from build123d import *

# Parameters (mm, degrees)
SKETCH1_R           = 10
BOSS_EXTRUDE1_DEPTH = 5
BOSS_EXTRUDE2_DEPTH = 125
SKETCH3_W           = 50
SKETCH3_H           = 35
CUT_EXTRUDE1_DEPTH  = 30
FILLET1_R           = 5
CHAMFER1_SIZE       = 0.5


with BuildPart() as part:
    # Sketch1 → Boss-Extrude1 (new body)
    with BuildSketch(Plane(origin=(0, 0, 0), x_dir=(1, 0, 0), z_dir=(0, 1, 0))):
        with BuildLine():
            Line((-105, 150), (105, 150))
            ThreePointArc((105, 150), (119.142135624, 144.142135624), (125, 130))
            Line((125, 130), (125, 0))
            Line((125, 0), (-125, 0))
            Line((-125, 0), (-125, 130))
            ThreePointArc((-125, 130), (-119.142135624, 144.142135624), (-105, 150))
        make_face()
        with Locations(Location((-85, 75, 0), (0, 0, 270))):
            Circle(SKETCH1_R, mode=Mode.SUBTRACT)
        with Locations(Location((85, 75, 0), (0, 0, 270))):
            Circle(SKETCH1_R, mode=Mode.SUBTRACT)
        with Locations(Location((0, 120, 0), (0, 0, 270))):
            Circle(SKETCH1_R, mode=Mode.SUBTRACT)
    extrude(amount=BOSS_EXTRUDE1_DEPTH)

    # Sketch2 → Boss-Extrude2 (add, symmetric)
    with BuildSketch(Plane(origin=(0, 0, 0), x_dir=(0, 0, -1), z_dir=(1, 0, 0))):
        with BuildLine():
            Line((0, 0), (-15, 0))
            ThreePointArc((-15, 0), (-22.745966692, 27.845232579), (-1.733500839, 8))
            Line((-1.733500839, 8), (-4.091287885, 8))
            ThreePointArc((-4.091287885, 8), (-5.774538708, 8.91987655), (-5.909406571, 10.833333333))
            ThreePointArc((-5.909406571, 10.833333333), (-20.400617249, 23.416254115), (-15, 5))
            Line((-15, 5), (0, 5))
            Line((0, 5), (0, 0))
        make_face()
    extrude(amount=BOSS_EXTRUDE2_DEPTH, both=True)

    # Sketch3 → Cut-Extrude1 (cut, symmetric)
    with BuildSketch(Plane(origin=(0, 0, 0), x_dir=(1, 0, 0), z_dir=(0, 1, 0))):
        with Locations((-100, -12.5)):
            Rectangle(SKETCH3_W, SKETCH3_H)
        with Locations((0, -12.5)):
            Rectangle(SKETCH3_W, SKETCH3_H)
        with Locations((100, -12.5)):
            Rectangle(SKETCH3_W, SKETCH3_H)
    extrude(amount=CUT_EXTRUDE1_DEPTH, both=True, mode=Mode.SUBTRACT)

    # Fillet1
    fillet1_edges = [part.edges().sort_by_distance(p)[0] for p in [
        (75, 2.5, -5),
        (-75, 2.5, -5),
        (25, 2.5, -5),
        (-25, 2.5, -5),
    ]]
    fillet(fillet1_edges, radius=FILLET1_R)

    # Chamfer1
    chamfer1_edges = [part.edges().sort_by_distance(p)[0] for p in [
        (-85, 0, -85),
        (-85, 5, -85),
        (85, 0, -85),
        (85, 5, -85),
        (0, 0, -130),
        (0, 5, -130),
    ]]
    chamfer(chamfer1_edges, length=CHAMFER1_SIZE)


solid = part.part
Here's how the part is built. I have some questions about the finished solid (model axes, mm). A direction names the side the tool comes from. Round coordinates to 2 decimals unless told otherwise and drop trailing zeros. Write each loop counter-clockwise with the first axis right and the second up, starting at its lowest first coordinate (ties: lowest second). Pieces come first, ordered by that corner, then holes.
1. For faces 1 (the flat face through (-75, 11, 5)), 2 (the cylindrical face through (23, 2, -4)), 3 (the flat face through (75, 12, 5)), which set-ups out of +Z, -Z, +X, -X, +Y, -Y let a thin tool reach every point of the face, with its end or its side?
2. Will these pins go through, and if not, where does the flat tip stop? pin 1 Ø4 at (x, y) = (-31, 22) entering from +Z; pin 2 Ø3 at (x, z) = (43, -118.5) entering from +Y; pin 3 Ø8 at (x, y) = (31.5, 22) entering from -Z; pin 4 Ø6 at (x, z) = (-23.5, -42.5) entering from -Y.
3. If we mould it in two halves opening along Y, with no side actions, what happens to faces 4 (the flat face through (2, 0, -69)), 5 (the cylindrical face through (-49.6, 23.6, 20.1)), 6 (the flat face through (0, 2, -5))? For each: released by +Y, released by -Y, zero draft, split by the parting line, or undercut.
4. I need wall thicknesses on L1, parallel to X at y = 3, z = -75; L2, parallel to Z at x = 58, y = 15; L3, parallel to X at y = 3.35, z = -120. Which ranges of each line are inside material? Lowest first, please.
5. Suppose I cut it at B-B (z = -120). List the corners of the cut face in (x, y) for me.
6. Suppose I cut it at D-D (z = -75). List the corners of the cut face in (x, y) for me, and give its area (3 significant figures).
7. Suppose I cut it at C-C (y = 27.5). List the corners of the cut face in (x, z) for me.
8. Suppose I cut it at A-A (x = 0). List the corners of the cut face in (y, z) for me, and give its area (4 significant figures).
Answer sheet:
1. face 1: +Z, -X, +Y, -Y
1. face 2: +Z, +Y, -Y
1. face 3: +Z, +X, +Y, -Y
2. pin 1: stops at z = 29.14
2. pin 2: stops at y = 5
2. pin 3: stops at z = 0.3
2. pin 4: stops at y = 0
3. face 4: released by -Y
3. face 5: undercut
3. face 6: zero draft
4. L1: x = -125 to -95, -75 to 75, 95 to 125
4. L2: z = 0 to 5, 25 to 30
4. L3: x = -125 to -10, 10 to 125
5. outline: (-125, 0) - (-10.5, 0) - (-10, 0.5) - (-10, 4.5) - (-10.5, 5) - (-125, 5) - close; (10, 0.5) - (10.5, 0) - (125, 0) - (125, 5) - (10.5, 5) - (10, 4.5) - close
6. outline: (-125, 0) - (-95.5, 0) - (-95, 0.5) - (-95, 4.5) - (-95.5, 5) - (-125, 5) - close; (-75, 0.5) - (-74.5, 0) - (74.5, 0) - (75, 0.5) - (75, 4.5) - (74.5, 5) - (-74.5, 5) - (-75, 4.5) - close; (95, 0.5) - (95.5, 0) - (125, 0) - (125, 5) - (95.5, 5) - (95, 4.5) - close
6. area: 1,050 mm2
7. outline: (-75, 6.71) - (-25, 6.71) - (-25, 23.29) - (-75, 23.29) - close; (25, 6.71) - (75, 6.71) - (75, 23.29) - (25, 23.29) - close
8. outline: (0, -150) - (5, -150) - (5, -130.5) - (4.5, -130) - (0.5, -130) - (0, -130.5) - close; (0, -109.5) - (0.5, -110) - (4.5, -110) - (5, -109.5) - (5, -5) - (0, -5) - close
8. area: 624.5 mm2
